Part model, mm, in its own coordinate system. Give positions to 0.01 mm unless a question says otherwise; leave off trailing zeros. Write each loop counter-clockwise with the first axis right and the second up, starting at its lowest first coordinate (ties: lowest second). Pieces come first, ordered by that corner, then holes.
from build123d import *

# Parameters (mm, degrees)
SKETCH2_W             = 50.8
SKETCH2_H             = 19.05
BOSS_EXTRUDE1_DEPTH   = 3.96875
F_8_CLEARANCE_HOLE1_D = 4.3053
CHAMFER1_SIZE         = 1.6002


with BuildPart() as part:
    # Sketch2 → Boss-Extrude1 (new body)
    with BuildSketch(Plane.XY):
        Rectangle(SKETCH2_W, SKETCH2_H)
    extrude(amount=BOSS_EXTRUDE1_DEPTH)

    # #8 Clearance Hole1 (through all)
    with Locations(Plane.XY.offset(3.96875)):
        with Locations((-17.4625, 0), (17.4625, 0)):
            Hole(F_8_CLEARANCE_HOLE1_D / 2)

    # Chamfer1
    chamfer1_edges = [part.edges().sort_by_distance(p)[0] for p in [
        (-25.4, 0, 3.96875),
        (0, -9.525, 3.96875),
        (25.4, 0, 3.96875),
        (0, 9.525, 3.96875),
    ]]
    chamfer(chamfer1_edges, length=CHAMFER1_SIZE)


solid = part.part
1) Saw through at C-C (x = 1.5). Write the cut outline in (y, z) (3 decimals), and give its area (3 significant figures).
Check result:
outline: (-9.525, 0) - (9.525, 0) - (9.525, 2.369) - (7.925, 3.969) - (-7.925, 3.969) - (-9.525, 2.369) - close
area: 73.0 mm2
2) Flat gauge pins, fed straight in: P1, Ø3.5, axis at x = 17.46, y = 0, coming from the +Z side; P2, Ø1, axis at y = 6.5, z = 3.5, coming from the -X side; P3, Ø1, axis at y = 0, z = 3, coming from the +X side. Where does each tip first touch, or does it go through?
Check result:
P1: passes through
P2: stops at x = -24.77
P3: stops at x = 25.27
3) Drill centre lines: L1, parallel to X at y = -0.25, z = 1.05; L2, parallel to Y at x = 17.5, z = 1.9 (3 decimals); L3, parallel to Y at x = 18.5, z = 1.25 (3 decimals). Where is each one in solid material? Low to high.
Check result:
L1: x = -25.4 to -19.6, -15.32 to 15.32, 19.6 to 25.4
L2: y = -9.525 to -2.152, 2.152 to 9.525
L3: y = -9.525 to -1.886, 1.886 to 9.525
4) Saw through at A-A (y = 0). Write the cut outline in (x, z), and give its area (3 significant figures).
Check result:
outline: (-25.4, 0) - (-19.62, 0) - (-19.62, 3.97) - (-23.8, 3.97) - (-25.4, 2.37) - close; (-15.31, 0) - (15.31, 0) - (15.31, 3.97) - (-15.31, 3.97) - close; (19.62, 0) - (25.4, 0) - (25.4, 2.37) - (23.8, 3.97) - (19.62, 3.97) - close
area: 165 mm2
5) Mould opens along X. For faces 1 (the cylindrical face through (15.41, 0.65, 1.96)), 2 (the flat face through (-24.59, -0.13, 3.18)), 3 (the flat face through (0, -9.525, 1)), 4 (the flat face through (25.4, 0, 1)) say: +X half, -X half, draft (parallel to the pull), parting line (faces both ways), or undercut.
Check result:
face 1: undercut
face 2: -X half
face 3: draft
face 4: +X half
6) Saw through at D-D (z = 3.4). Write the cut outline in (x, y), and give its area (3 significant figures).
Check result:
outline: (-24.37, -8.49) - (24.37, -8.49) - (24.37, 8.49) - (-24.37, 8.49) - close; hole circle Ø4.31 at (-17.46, 0); hole circle Ø4.31 at (17.46, 0)
area: 799 mm2
7) Saw through at B-B (z = 0.5). Write the cut outline in (x, y) (1 decimal), and give its area (3 significant figures).
Check result:
outline: (-25.4, -9.5) - (25.4, -9.5) - (25.4, 9.5) - (-25.4, 9.5) - close; hole circle Ø4.3 at (-17.5, 0); hole circle Ø4.3 at (17.5, 0)
area: 939 mm2
